```python
from build123d import *

# Parameters (mm, degrees)
SKETCH_2_W          = 96.5
SKETCH_2_H          = 18
EXTRUDE_1_DEPTH     = 12
SKETCH_3_W          = 14
SKETCH_3_H          = 14
CUT_EXTRUDE_1_DEPTH = 1.2
SKETCH_4_W          = 56
SKETCH_4_H          = 15
CUT_EXTRUDE_2_DEPTH = 4.8
CHAMFER_1_SIZE      = 0.3
CHAMFER_2_SIZE      = 3
SKETCH_6_W          = 6
SKETCH_6_H          = 4
CUT_EXTRUDE_3_DEPTH = 99.895146494
CUT_EXTRUDE_START   = -4
SKETCH_6_4_W        = 6
SKETCH_6_4_H        = 6.1
CUT_EXTRUDE_5_DEPTH = 95.895146494
SKETCH_7_W          = 69.4
SKETCH_7_H          = 10
CUT_EXTRUDE_4_DEPTH = 6
CHAMFER_3_SIZE      = 0.4
SKETCH_8_R          = 1.2
CUT_EXTRUDE_6_DEPTH = 99.245865053
SKETCH_9_R          = 2.05
CUT_EXTRUDE_7_DEPTH = 2
SKETCH_9_3_R        = 1.2
CUT_EXTRUDE_8_DEPTH = 99.895146494
CHAMFER_4_SIZE      = 1
CHAMFER_5_SIZE      = 2
CHAMFER_6_SIZE      = 0.8
CHAMFER_7_SIZE      = 1


with BuildPart() as part:
    # 草图2 → 凸台-拉伸1 (new body)
    with BuildSketch(Plane(origin=(0, 0, 0), x_dir=(0, 0, -1), z_dir=(1, 0, 0))):
        with Locations((48.25, 9)):
            Rectangle(SKETCH_2_W, SKETCH_2_H)
    extrude(amount=EXTRUDE_1_DEPTH)

    # 草图3 → 切除-拉伸1 (cut)
    with BuildSketch(Plane(origin=(12, 0, 0), x_dir=(0, 0, -1), z_dir=(1, 0, 0))):
        with Locations((85, 9)):
            Rectangle(SKETCH_3_W, SKETCH_3_H)
        with Locations((66, 9)):
            Rectangle(SKETCH_3_W, SKETCH_3_H)
        with Locations((47, 9)):
            Rectangle(SKETCH_3_W, SKETCH_3_H)
    extrude(amount=-CUT_EXTRUDE_1_DEPTH, mode=Mode.SUBTRACT)

    # 草图4 → 切除-拉伸2 (cut)
    with BuildSketch(Plane(origin=(10.8, 0, 0), x_dir=(0, 0, -1), z_dir=(1, 0, 0))):
        with Locations((64.5, 9)):
            Rectangle(SKETCH_4_W, SKETCH_4_H)
    extrude(amount=-CUT_EXTRUDE_2_DEPTH, mode=Mode.SUBTRACT)

    # 倒角1
    chamfer_1_edges = [part.edges().sort_by_distance(p)[0] for p in [
        (10.8, 1.5, -64.5),
        (10.8, 16.5, -64.5),
    ]]
    chamfer(chamfer_1_edges, length=CHAMFER_1_SIZE)

    # 倒角2
    chamfer_2_edges = [part.edges().sort_by_distance(p)[0] for p in [
        (6, 16.5, -64.5),
        (6, 1.5, -64.5),
    ]]
    chamfer(chamfer_2_edges, length=CHAMFER_2_SIZE)

    # 草图6 → 切除-拉伸3 (cut, through all)
    with BuildSketch(Plane(origin=(0, 0, -96.5), x_dir=(-1, 0, 0), z_dir=(0, 0, -1))):
        with Locations((-3, 16)):
            Rectangle(SKETCH_6_W, SKETCH_6_H)
        with Locations((-3, 2)):
            Rectangle(SKETCH_6_W, SKETCH_6_H)
    extrude(amount=-CUT_EXTRUDE_3_DEPTH, mode=Mode.SUBTRACT)

    # 草图6<4> → 切除-拉伸5 (cut, through all)
    with BuildSketch(Plane(origin=(0, 0, -96.5), x_dir=(-1, 0, 0), z_dir=(0, 0, -1)).offset(CUT_EXTRUDE_START)):
        with Locations((-3, 9)):
            Rectangle(SKETCH_6_4_W, SKETCH_6_4_H)
    extrude(amount=-CUT_EXTRUDE_5_DEPTH, mode=Mode.SUBTRACT)

    # 草图7 → 切除-拉伸4 (cut)
    with BuildSketch(Plane.ZY):
        with Locations((-57.8, 9)):
            Rectangle(SKETCH_7_W, SKETCH_7_H)
    extrude(amount=-CUT_EXTRUDE_4_DEPTH, mode=Mode.SUBTRACT)

    # 倒角3
    chamfer_3_edges = [part.edges().sort_by_distance(p)[0] for p in [
        (0, 4.975, 0),
        (0, 9, -92.5),
        (3, 12.05, -23.1),
        (0, 13.025, -23.1),
        (3, 5.95, -23.1),
        (0, 4.975, -23.1),
        (0, 13.025, 0),
        (0, 9, -96.5),
    ]]
    chamfer(chamfer_3_edges, length=CHAMFER_3_SIZE)

    # 草图8 → 切除-拉伸6 (cut, through all)
    with BuildSketch(Plane(origin=(0, 14, 0), x_dir=(1, 0, 0), z_dir=(0, 1, 0))):
        with Locations(Location((3.2, 17.25, 0), (0, 0, 270))):
            Circle(SKETCH_8_R)
    extrude(amount=-CUT_EXTRUDE_6_DEPTH, mode=Mode.SUBTRACT)

    # 草图9 → 切除-拉伸7 (cut)
    with BuildSketch(Plane(origin=(0, 0, -96.5), x_dir=(-1, 0, 0), z_dir=(0, 0, -1))):
        with Locations((-3, 9)):
            Circle(SKETCH_9_R)
    extrude(amount=-CUT_EXTRUDE_7_DEPTH, mode=Mode.SUBTRACT)

    # 草图9<3> → 切除-拉伸8 (cut, through all)
    with BuildSketch(Plane(origin=(0, 0, -96.5), x_dir=(-1, 0, 0), z_dir=(0, 0, -1))):
        with Locations((-3, 9)):
            Circle(SKETCH_9_3_R)
    extrude(amount=-CUT_EXTRUDE_8_DEPTH, mode=Mode.SUBTRACT)

    # 倒角4
    chamfer_4_edges = [part.edges().sort_by_distance(p)[0] for p in [
        (6, 18, -48.25),
        (6, 0, -48.25),
        (12, 9, -96.5),
        (9, 18, -96.5),
        (9, 0, -96.5),
    ]]
    chamfer(chamfer_4_edges, length=CHAMFER_4_SIZE)

    # 倒角5
    chamfer_5_edges = [part.edges().sort_by_distance(p)[0] for p in [
        (12, 9, 0),
    ]]
    chamfer(chamfer_5_edges, length=CHAMFER_5_SIZE)

    # 倒角6
    chamfer_6_edges = [part.edges().sort_by_distance(p)[0] for p in [
        (12, 18, -48.75),
        (12, 0, -48.75),
    ]]
    chamfer(chamfer_6_edges, length=CHAMFER_6_SIZE)

    # 倒角7
    chamfer_7_edges = [part.edges().sort_by_distance(p)[0] for p in [
        (8.5, 0, 0),
        (8.5, 18, 0),
    ]]
    chamfer(chamfer_7_edges, length=CHAMFER_7_SIZE)


solid = part.part
```
The model under review builds one solid part; all positions refer to its coordinate system, in mm. A direction names the side the tool comes from. Give positions to 0.01 mm unless a question says otherwise; leave off trailing zeros. Write each loop counter-clockwise with the first axis right and the second up, starting at its lowest first coordinate (ties: lowest second). Pieces come first, ordered by that corner, then holes. Notation, with made-up numbers: M 29,66 L 44,66 A17 ccw 44,73 Z; hole C -28,11.5 d10. An arc over 180 degrees is marked long. Answer in a Markdown table with one row per item.
Item 1: Add section D-D on z = -7. Give the boundary of the cut face in (x, y), plus the area to 3 significant figures.
Check sheet entries:
| item | result |
|---|---|
| outline | M 0,4 L 6,4 L 6,1 L 7,0 L 11.2,0 L 12,0.8 L 12,17.2 L 11.2,18 L 7,18 L 6,17 L 6,14 L 0,14 L 0,12.05 L 6,12.05 L 6,5.95 L 0,5.95 Z |
| area | 130 mm2 |
Item 2: For P1, Ø1.3, axis at x = 11.5, y = 10.5, coming from the +Z side; P2, Ø3, axis at x = 3, z = -9.5, coming from the -Y side; P3, Ø1, axis at x = 11.5, y = 5.5, coming from the +Z side, all flat-tipped, find the tip position at first contact; note any pin that passes through.
Check sheet entries:
| item | result |
|---|---|
| P1 | z = -0.85 |
| P2 | y = 4 |
| P3 | z = -1 |
Item 3: For line 1 along Y through (x, z) = (2.75, -5.5); line 2 along X through (y, z) = (5.5, -17.25); line 3 along Z through (x, y) = (9.25, 3.5), list the stretches that pass through material, from the lowest coordinate up.
Check sheet entries:
| item | result |
|---|---|
| line 1 | 4 to 5.95, 12.05 to 14 |
| line 2 | 0 to 2, 4.4 to 12 |
| line 3 | -96.5 to -92.5, -36.5 to 0 |
Item 4: Add section A-A on y = 9. State how many separate pieces and enclosed holes the cut face has, plus the area to 3 significant figures.
Check sheet entries:
| item | result |
|---|---|
| separate pieces | 5 |
| enclosed holes | 0 |
| area | 268 mm2 |
Item 5: Draft analysis for pull direction Y (two halves, no side actions). For faces 4 (the face through (3, 5, -23.1)), 5 (the face through (8, 9, -36.5)), 6 (the face through (10, 16.5, -64)), 7 (the face through (9, 18, -48)), state which applies: +Y half, -Y half, draft (parallel to the pull), parting line (faces both ways), or undercut.
Check sheet entries:
| item | result |
|---|---|
| face 4 | draft |
| face 5 | undercut |
| face 6 | undercut |
| face 7 | +Y half |
Item 6: Tool access review of faces 1 (the face through (3, 5.95, -12)), 2 (the face through (2, 8, -94.5)), 3 (the face through (10.8, 9, -58)): name each direction out of +Z, -Z, +X, -X, +Y, -Y from which nothing blocks a thin tool from reaching the whole face with its end or side.
Check sheet entries:
| item | result |
|---|---|
| face 1 | +Z, -X |
| face 2 | -Z |
| face 3 | none |
Item 7: Add section C-C on z = -61. Give the boundary of the cut face in (x, y).
Check sheet entries:
| item | result |
|---|---|
| outline | M 6,1 L 7,0 L 11.2,0 L 12,0.8 L 12,2 L 10.8,2 L 10.8,1.8 L 10.5,1.5 L 9,1.5 L 6,4.5 Z; M 6,13.5 L 9,16.5 L 10.5,16.5 L 10.8,16.2 L 10.8,16 L 12,16 L 12,17.2 L 11.2,18 L 7,18 L 6,17 Z |
Item 8: Add section B-B on z = -17.25. Give the boundary of the cut face in (x, y).
Check sheet entries:
| item | result |
|---|---|
| outline | M 0,4 L 2,4 L 2,5.95 L 0,5.95 Z; M 0,12.05 L 2,12.05 L 2,14 L 0,14 Z; M 4.4,4 L 6,4 L 6,1 L 7,0 L 11.2,0 L 12,0.8 L 12,17.2 L 11.2,18 L 7,18 L 6,17 L 6,14 L 4.4,14 L 4.4,12.05 L 6,12.05 L 6,5.95 L 4.4,5.95 Z |
